Check sheet for the drawn part. Datum: minimum x, y, z corner. Units: mm. Round coordinates to 2 decimals unless told otherwise and drop trailing zeros. Write each loop counter-clockwise with the first axis right and the second up, starting at its lowest first coordinate (ties: lowest second). Pieces come first, ordered by that corner, then holes.
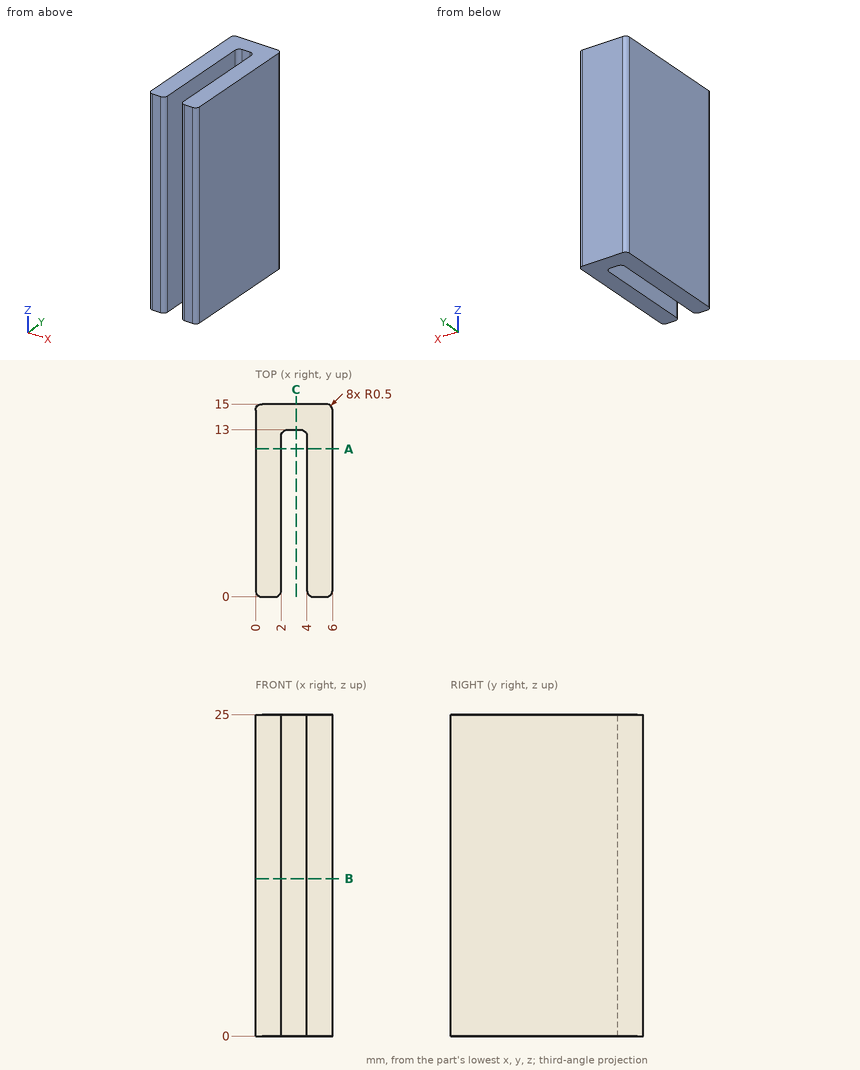
Q1. Sectioned sample at A-A (y = 11.5). Enter the section's corners in (x, z), plus the area to 3 significant figures.
Recorded:
outline: (0, 0) - (2, 0) - (2, 25) - (0, 25) - close; (4, 0) - (6, 0) - (6, 25) - (4, 25) - close
area: 100 mm2
Q2. Sectioned sample at C-C (x = 3.15). Enter the section's corners in (y, z), plus the area to 3 significant figures.
Recorded:
outline: (13, 0) - (15, 0) - (15, 25) - (13, 25) - close
area: 50.0 mm2
Q3. Material ranges on line 1 along X through (y, z) = (5, 14.75); line 2 along Y through (x, z) = (3.15, 21); line 3 along X through (y, z) = (12.75, 2.25), recorded low to high.
Recorded:
line 1: x = 0 to 2, 4 to 6
line 2: y = 13 to 15
line 3: x = 0 to 2.07, 3.93 to 6
Q4. Depth check by flat-ended pin: P1, Ø0.8, axis at x = 3, z = 9, coming from the -Y side. Enter the tip coordinate at first touch or a pass-through.
Recorded:
P1: stops at y = 13
Q5. Sectioned sample at B-B (z = 12.25). Enter the section's corners in (x, y).
Recorded:
outline: (0, 0.5) arc R0.5 ccw to (0.5, 0) - (1.5, 0) arc R0.5 ccw to (2, 0.5) - (2, 12.5) arc R0.5 cw to (2.5, 13) - (3.5, 13) arc R0.5 cw to (4, 12.5) - (4, 0.5) arc R0.5 ccw to (4.5, 0) - (5.5, 0) arc R0.5 ccw to (6, 0.5) - (6, 14.5) arc R0.5 ccw to (5.5, 15) - (0.5, 15) arc R0.5 ccw to (0, 14.5) - close
